Check sheet for the modelled part. Datum: model origin and axes. Units: mm. Face numbers are marked on the shaded views. A direction names the side the tool comes from. Give positions to 0.01 mm unless a question says otherwise; leave off trailing zeros. Order: outer loops, then holes, each group sorted by start corner. A loop starts at its lowest first (then second) coordinate and runs counter-clockwise, first axis right, second up.
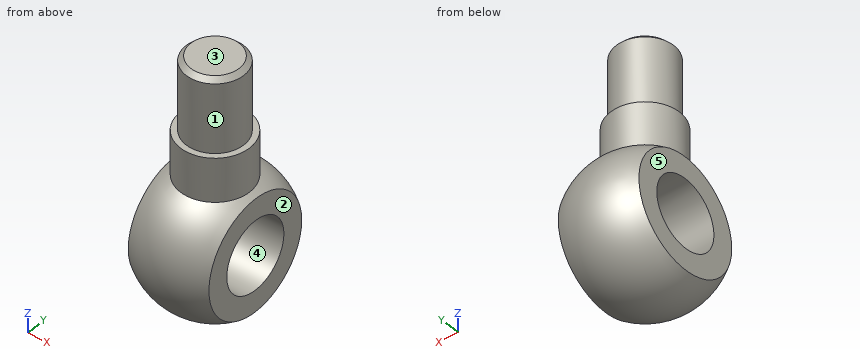
from build123d import *

# Parameters (mm, degrees)
P_IDAT_VYSUNUT_M1_REACH = 77
SKICA4_R                = 15
SKICA5_R                = 12.5
P_IDAT_VYSUNUT_M2_DEPTH = 32
ZKOSEN_1_SIZE           = 2


with BuildPart() as part:
    # Skica1 → Rotovat1 (revolve)
    with BuildSketch(Plane.XY):
        with BuildLine():
            ThreePointArc((17.5, 24.366985862), (0, 30), (-17.5, 24.366985862))
            Line((-17.5, 24.366985862), (-17.5, 15))
            Line((-17.5, 15), (17.5, 15))
            Line((17.5, 15), (17.5, 24.366985862))
        make_face()
    revolve(axis=Axis((-37.473333333, 0, 0), (1, 0, 0)))

    # Skica4 → Přidat vysunutím1 (add, up to next)
    with BuildSketch(Plane.XY.offset(45), mode=Mode.PRIVATE) as p_idat_vysunut_m1_sk1:
        Circle(SKICA4_R)
    p_idat_vysunut_m1_tool1 = extrude(p_idat_vysunut_m1_sk1.sketch, amount=-P_IDAT_VYSUNUT_M1_REACH, mode=Mode.PRIVATE) - part.part
    add(p_idat_vysunut_m1_tool1.solids().sort_by_distance((0, 0, 45))[0])

    # Skica5 → Přidat vysunutím2 (add)
    with BuildSketch(Plane.XY.offset(45)):
        Circle(SKICA5_R)
    extrude(amount=P_IDAT_VYSUNUT_M2_DEPTH)

    # Zkosení1
    zkosen_1_edges = [part.edges().sort_by_distance(p)[0] for p in [
        (-12.5, 0, 77),
    ]]
    chamfer(zkosen_1_edges, length=ZKOSEN_1_SIZE)


solid = part.part
1) Material ranges on L1, parallel to Z at x = -8, y = 13; L2, parallel to Y at x = -11, z = 5.5; L3, parallel to Z at x = 9, y = 0, recorded low to high.
Recorded:
L1: z = -25.83 to -7.48, 7.48 to 25.83
L2: y = -27.36 to -13.96, 13.96 to 27.36
L3: z = -28.62 to -15, 15 to 77
2) Draft check along Z on the marked faces 3, 4 and 5. Enter one of: +Z half, -Z half, draft (parallel to the pull), parting line (faces both ways), or undercut.
Recorded:
face 3: +Z half
face 4: undercut
face 5: draft
3) Depth check by flat-ended pin: pin 1 Ø4 at (x, y) = (-8, -15.5) entering from +Z; pin 2 Ø1 at (x, z) = (13.5, 33.5) entering from -Y; pin 3 Ø4 at (x, z) = (4, 60) entering from -Y. Enter the tip coordinate at first touch or a pass-through.
Recorded:
pin 1: stops at z = 25.72
pin 2: stops at y = -7.48
pin 3: stops at y = -12.34
4) Section check B-B, the plane y = 0. Record the cut outline in (x, z).
Recorded:
outline: (-17.5, -24.37) arc R30 ccw to (17.5, -24.37) - (17.5, -15) - (-17.5, -15) - close; (-17.5, 15) - (17.5, 15) - (17.5, 24.37) arc R30 ccw to (15, 25.98) - (15, 45) - (12.5, 45) - (12.5, 75) - (10.5, 77) - (-10.5, 77) - (-12.5, 75) - (-12.5, 45) - (-15, 45) - (-15, 25.98) arc R30 ccw to (-17.5, 24.37) - close
5) Section check D-D, the plane z = 33. Record the cut outline in (x, y), then the cut area to 3 significant figures.
Recorded:
outline: circle Ø30 at (0, 0)
area: 707 mm2
6) Section check A-A, the plane x = 0. Record the cut outline in (y, z), then the cut area to 3 significant figures.
Recorded:
outline: (-15, 25.98) arc R30 ccw (long way) to (15, 25.98) - (15, 45) - (12.5, 45) - (12.5, 75) - (10.5, 77) - (-10.5, 77) - (-12.5, 75) - (-12.5, 45) - (-15, 45) - close; hole circle Ø30 at (0, 0)
area: 3,410 mm2
7) Section check C-C, the plane z = 0. Record the cut outline in (x, y).
Recorded:
outline: (-17.5, -24.37) arc R30 ccw to (17.5, -24.37) - (17.5, -15) - (-17.5, -15) - close; (-17.5, 15) - (17.5, 15) - (17.5, 24.37) arc R30 ccw to (-17.5, 24.37) - close
8) Set-up check for the marked faces 1 and 2: record each of +Z, -Z, +X, -X, +Y, -Y from which the full face is reachable in a straight line by a thin tool's end or side.
Recorded:
face 1: +Z
face 2: +Z, -Z, +X, +Y, -Y
